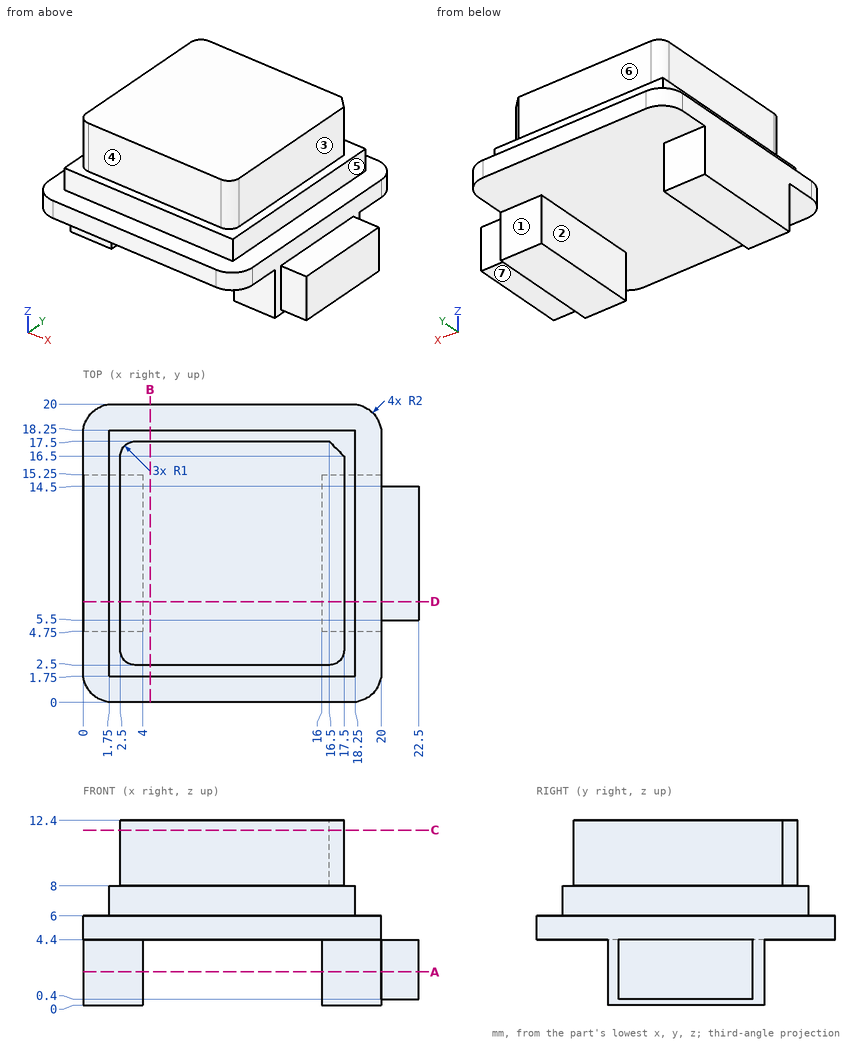
Job drawing, mm, ordinate dimensions from the low corner. One solid piece. A direction names the side the tool comes from. Round coordinates to 2 decimals unless told otherwise and drop trailing zeros. Loops run counter-clockwise (first coordinate to the right, second up) from the corner with the lowest first, then second, coordinate; pieces in that order, holes last. Notation, with made-up numbers: (40.25, 7.25) -> (74.25, 7.25) arc R15 cw to (74.25, 19.25) -> close; hole circle Ø11 at (-34, -14). An arc over 180 degrees is marked (long way). Use CSV: the item, a comma, the result in double quotes. Start each with the question number.
Q1. Drill centre lines: L1, parallel to X at y = 10, z = 8.75; L2, parallel to Z at x = 4, y = 3.5; L3, parallel to Z at x = 12.75, y = 19. Where is each one in solid material? Low to high.
Q2. Saw through at B-B on x = 4.5. Give the cut face in (y, z).
Q3. Flat gauge pins, fed straight in: pin 1 Ø4 at (x, y) = (9, 9) entering from -Z; pin 2 Ø2 at (x, z) = (1, 1.5) entering from +Y; pin 3 Ø5 at (y, z) = (11, 9) entering from -X. Where does each tip first touch, or does it go through?
Q4. Mould opens along X. For the marked faces 1, 2 and 3 say: +X half, -X half, draft (parallel to the pull), parting line (faces both ways), or undercut.
Q5. Which spindle directions (+Z, -Z, +X, -X, +Y, -Y) get a long thin tool onto all of the face, cutting with end or side? Do the marked faces 4, 5, 6 and 7. Say none if no direction does.
Q6. Saw through at C-C on z = 11.75. Give the cut face in (x, y), and give its area (3 significant figures).
Q7. Saw through at D-D on y = 6.75. Give the cut face in (x, z).
Q8. Saw through at A-A on z = 2.25. Give the cut face in (x, y), and give its area (4 significant figures).
Solutions:
1,L1,"x = 2.5 to 17.5"
1,L2,"z = 4.4 to 12.4"
1,L3,"z = 4.4 to 6"
2,outline,"(0, 4.4) -> (20, 4.4) -> (20, 6) -> (18.25, 6) -> (18.25, 8) -> (17.5, 8) -> (17.5, 12.4) -> (2.5, 12.4) -> (2.5, 8) -> (1.75, 8) -> (1.75, 6) -> (0, 6) -> close"
3,pin 1,"stops at z = 4.4"
3,pin 2,"stops at y = 15.25"
3,pin 3,"stops at x = 1.75"
4,face 1,"draft"
4,face 2,"undercut"
4,face 3,"+X half"
5,face 4,"+Z, +X, -X, -Y"
5,face 5,"+Z, +X, +Y, -Y"
5,face 6,"+Z, +X, -X, +Y"
5,face 7,"-Z, +X, +Y, -Y"
6,outline,"(2.5, 3.5) arc R1 ccw to (3.5, 2.5) -> (16.5, 2.5) arc R1 ccw to (17.5, 3.5) -> (17.5, 16.5) -> (16.5, 17.5) -> (3.5, 17.5) arc R1 ccw to (2.5, 16.5) -> close"
6,area,"224 mm^2"
7,outline,"(0, 0) -> (4, 0) -> (4, 4.4) -> (16, 4.4) -> (16, 0) -> (20, 0) -> (20, 0.4) -> (22.5, 0.4) -> (22.5, 4.4) -> (20, 4.4) -> (20, 6) -> (18.25, 6) -> (18.25, 8) -> (17.5, 8) -> (17.5, 12.4) -> (2.5, 12.4) -> (2.5, 8) -> (1.75, 8) -> (1.75, 6) -> (0, 6) -> close"
8,outline,"(0, 4.75) -> (4, 4.75) -> (4, 15.25) -> (0, 15.25) -> close; (16, 4.75) -> (20, 4.75) -> (20, 5.5) -> (22.5, 5.5) -> (22.5, 14.5) -> (20, 14.5) -> (20, 15.25) -> (16, 15.25) -> close"
8,area,"106.5 mm^2"
